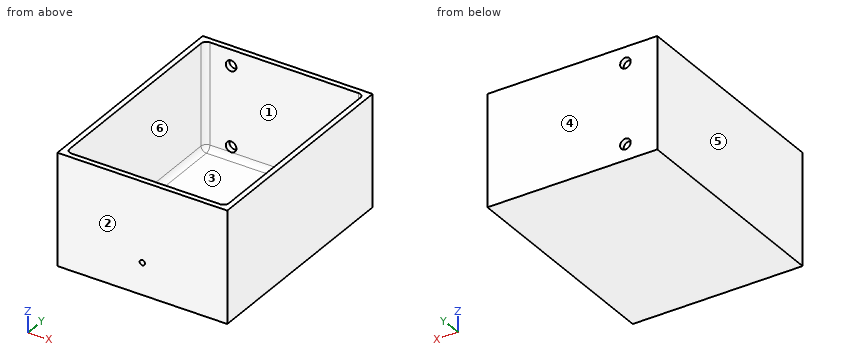
```python
from build123d import *

# Parameters (mm, degrees)
SKETCH1_W           = 160
SKETCH1_H           = 210
SKETCH1_W_2         = 150
SKETCH1_H_2         = 200
BOSS_EXTRUDE1_DEPTH = 100
SKETCH3_W           = 160
SKETCH3_H           = 210
BOSS_EXTRUDE2_DEPTH = 5
FILLET1_R           = 5
SKETCH4_R           = 5
CUT_EXTRUDE1_DEPTH  = 48
SKETCH5_R           = 2.5
CUT_EXTRUDE2_DEPTH  = 40


with BuildPart() as part:
    # Sketch1 → Boss-Extrude1 (new body)
    with BuildSketch(Plane.XY):
        Rectangle(SKETCH1_W, SKETCH1_H)
        Rectangle(SKETCH1_W_2, SKETCH1_H_2, mode=Mode.SUBTRACT)
    extrude(amount=BOSS_EXTRUDE1_DEPTH)

    # Sketch3 → Boss-Extrude2 (add)
    with BuildSketch(Plane(origin=(0, 0, 0), x_dir=(-1, 0, 0), z_dir=(0, 0, -1))):
        Rectangle(SKETCH3_W, SKETCH3_H)
    extrude(amount=BOSS_EXTRUDE2_DEPTH)

    # Fillet1
    fillet1_edges = [part.edges().sort_by_distance(p)[0] for p in [
        (-75, 0, 0),
        (-75, 100, 50),
        (0, -100, 0),
        (-75, -100, 50),
        (75, 0, 0),
        (75, -100, 50),
        (0, 100, 0),
        (75, 100, 50),
    ]]
    fillet(fillet1_edges, radius=FILLET1_R)

    # Sketch4 → Cut-Extrude1 (cut)
    with BuildSketch(Plane(origin=(0, 105, 0), x_dir=(1, 0, 0), z_dir=(0, 1, 0))):
        with Locations((-50, -10)):
            Circle(SKETCH4_R)
        with Locations((-50, -85)):
            Circle(SKETCH4_R)
    extrude(amount=-CUT_EXTRUDE1_DEPTH, mode=Mode.SUBTRACT)

    # Sketch5 → Cut-Extrude2 (cut)
    with BuildSketch(Plane.XZ.offset(105)):
        with Locations((0, 25)):
            Circle(SKETCH5_R)
    extrude(amount=-CUT_EXTRUDE2_DEPTH, mode=Mode.SUBTRACT)


solid = part.part
```
CAD build for the part. Positions are in the model's coordinates, mm. Face numbers are marked on the shaded views. A direction names the side the tool comes from. Round coordinates to 2 decimals unless told otherwise and drop trailing zeros. Loops run counter-clockwise (first coordinate to the right, second up) from the corner with the lowest first, then second, coordinate; pieces in that order, holes last. Notation, with made-up numbers: M 73,-3 L 111,-3 A31 ccw 111,32 Z; hole C 70.25,61.25 d8. An arc over 180 degrees is marked long. Use a Markdown table: item, result. Add a question column.
(1) Drill centre lines: line 1 (Z direction, x = -50, y = 101.9); line 2 (X direction, y = 37, z = 77); line 3 (Y direction, x = 44, z = 90.5). Where is each one in solid material? Low to high.
(2) Cut at D-D (z = 25). Give the cut face in (x, y), and give its area (3 significant figures).
(3) Flat gauge pin, fed straight in: pin 1 (4 mm diameter, centred on x = 0, z = 25, fed in from -Y). Where does the tip first touch, or does it go through?
(4) Cut at C-C (z = 66.5). Give the cut face in (x, y), and give its area (3 significant figures).
(5) Which spindle directions (+Z, -Z, +X, -X, +Y, -Y) get a long thin tool onto all of the face, cutting with end or side? Do the marked faces 1 and 2. Say none if no direction does.
(6) Cut at A-A (x = 0). Give the cut face in (y, z).
(7) Cut at B-B (y = 33). Give the cut face in (x, z).
(8) Pull direction X, two halves, no side cores. Call the marked faces 3, 4, 5 and 6: +X half, -X half, draft (parallel to the pull), parting line (faces both ways), or undercut.
Geometry says:
| question | item | result |
|---|---|---|
| 1 | line 1 | z = -5 to 5, 15 to 80, 90 to 100 |
| 1 | line 2 | x = -80 to -75, 75 to 80 |
| 1 | line 3 | y = -105 to -100, 100 to 105 |
| 2 | outline | M -80,-105 L -2.5,-105 L -2.5,-100 L -70,-100 A5 cw -75,-95 L -75,95 A5 cw -70,100 L 70,100 A5 cw 75,95 L 75,-95 A5 cw 70,-100 L 2.5,-100 L 2.5,-105 L 80,-105 L 80,105 L -80,105 Z |
| 2 | area | 3,600 mm² |
| 3 | pin 1 | stops at y = 100 |
| 4 | outline | M -80,-105 L 80,-105 L 80,105 L -80,105 Z; hole M -75,-95 A5 ccw -70,-100 L 70,-100 A5 ccw 75,-95 L 75,95 A5 ccw 70,100 L -70,100 A5 ccw -75,95 Z |
| 4 | area | 3,620 mm² |
| 5 | face 1 | +Z |
| 5 | face 2 | +Z, -Z, +X, -X, -Y |
| 6 | outline | M -105,-5 L 105,-5 L 105,100 L 100,100 L 100,5 A5 cw 95,0 L -95,0 A5 cw -100,5 L -100,22.5 L -105,22.5 Z; M -105,27.5 L -100,27.5 L -100,100 L -105,100 Z |
| 7 | outline | M -80,-5 L 80,-5 L 80,100 L 75,100 L 75,5 A5 cw 70,0 L -70,0 A5 cw -75,5 L -75,100 L -80,100 Z |
| 8 | face 3 | undercut |
| 8 | face 4 | draft |
| 8 | face 5 | -X half |
| 8 | face 6 | undercut |
